```python
from build123d import *

# Parameters (mm, degrees)
SKETCH_1_W           = 40
SKETCH_1_H           = 45
EXTRUDE_1_DEPTH      = 40
EXTRUDE_1_DEPTH_BACK = 5
SKETCH_2_W           = 36
SKETCH_2_H           = 37
CUT_EXTRUDE_1_DEPTH  = 50
SKETCH_3_R           = 1.025
CUT_EXTRUDE_2_DEPTH  = 2
SKETCH_4_R           = 1.025
CUT_EXTRUDE_3_DEPTH  = 2
SKETCH_5_W           = 36
SKETCH_5_H           = 5
CUT_EXTRUDE_4_DEPTH  = 43
FILLET_6_R           = 5
FILLET_7_R           = 5


with BuildPart() as part:
    # 草圖1 → 填料-伸長1 (new body, two sides)
    with BuildSketch(Plane.XY) as extrude_1_sk:
        with Locations((5.454545455, -5.590909091)):
            Rectangle(SKETCH_1_W, SKETCH_1_H)
    extrude(amount=EXTRUDE_1_DEPTH)
    extrude(extrude_1_sk.sketch, amount=-EXTRUDE_1_DEPTH_BACK)

    # 草圖2 → 除料-伸長1 (cut)
    with BuildSketch(Plane(origin=(0, 16.909090909, 0), x_dir=(1, 0, 0), z_dir=(0, 1, 0))):
        with Locations((5.454545455, -21.5)):
            Rectangle(SKETCH_2_W, SKETCH_2_H)
    extrude(amount=-CUT_EXTRUDE_1_DEPTH, mode=Mode.SUBTRACT)

    # 草圖3 → 除料-伸長2 (cut)
    with BuildSketch(Plane.ZY.offset(14.545454545)):
        with Locations((37, -25.090909091)):
            Circle(SKETCH_3_R)
        with Locations((37, 13.909090909)):
            Circle(SKETCH_3_R)
    extrude(amount=-CUT_EXTRUDE_2_DEPTH, mode=Mode.SUBTRACT)

    # 草圖4 → 除料-伸長3 (cut)
    with BuildSketch(Plane(origin=(25.454545455, 0, 0), x_dir=(0, 0, -1), z_dir=(1, 0, 0))):
        with Locations((-37, 13.909090909)):
            Circle(SKETCH_4_R)
        with Locations((-37, -25.090909091)):
            Circle(SKETCH_4_R)
    extrude(amount=-CUT_EXTRUDE_3_DEPTH, mode=Mode.SUBTRACT)

    # 草圖5 → 除料-伸長4 (cut)
    with BuildSketch(Plane(origin=(0, 16.909090909, 0), x_dir=(1, 0, 0), z_dir=(0, 1, 0))):
        with Locations((5.454545455, -0.5)):
            Rectangle(SKETCH_5_W, SKETCH_5_H)
    extrude(amount=-CUT_EXTRUDE_4_DEPTH, mode=Mode.SUBTRACT)

    # 圓角6
    fillet_6_edges = [part.edges().sort_by_distance(p)[0] for p in [
        (-14.545454545, -5.590909091, -5),
    ]]
    fillet(fillet_6_edges, radius=FILLET_6_R)

    # 圓角7
    fillet_7_edges = [part.edges().sort_by_distance(p)[0] for p in [
        (25.454545455, -5.590909091, -5),
    ]]
    fillet(fillet_7_edges, radius=FILLET_7_R)


solid = part.part
```
Could you check a few things on this model? Use its own coordinates, in mm. A direction names the side the tool comes from. Round coordinates to 2 decimals unless told otherwise and drop trailing zeros. Write each loop counter-clockwise with the first axis right and the second up, starting at its lowest first coordinate (ties: lowest second). Pieces come first, ordered by that corner, then holes. Notation, with made-up numbers: M 36,12 L 89,12 A14 ccw 89,33 Z; hole C 68.25,-37.75 d1. An arc over 180 degrees is marked long. Write each question's results on one line, items separated by ' | '. Start each with the question number.
1. Thinking about a two-plate mould opening in Y: for faces 4 (the face through (24.469, 13.954, 38.024)), 5 (the face through (5.4, -28.091, 2.6)), 6 (the face through (5, -26.091, 0)), which applies, +Y half, -Y half, draft (parallel to the pull), parting line (faces both ways), or undercut?
2. On a 3-axis mill with a long thin cutter (end or side, diameter ignored), from which of +Z, -Z, +X, -X, +Y, -Y can I reach the whole of each face in a straight line? I mean faces 1 (the face through (5, -4, -2)), 2 (the face through (5, -27, 3)), 3 (the face through (-13.12, -5.276, -3.496)). Say none if no direction works.
3. Imagine slicing it at B-B on z = 24.5. List the corners of the cut face in (x, y) for me.
4. Imagine slicing it at A-A on z = 37. List the corners of the cut face in (x, y) for me, and give its area (3 significant figures).
5. Imagine slicing it at D-D on x = 12. List the corners of the cut face in (y, z) for me, and give its area (3 significant figures).
6. I'm going to push flat-ended pins straight in: pin 1 Ø1.8 at (y, z) = (-25.09, 37) entering from +X; pin 2 Ø2.5 at (x, z) = (12.5, 1.5) entering from +Y; pin 3 Ø3.5 at (y, z) = (13.91, 37) entering from +X; pin 4 Ø3 at (x, y) = (9.5, 1.5) entering from +Z. Where does each tip first touch, or does it pass through?
7. Imagine slicing it at C-C on y = 8. List the corners of the cut face in (x, z) for me.
8. I need wall thicknesses on L1, parallel to Y at x = 23.95, z = 37; L2, parallel to X at y = -13, z = 0.5; L3, parallel to Z at x = 14, y = -25.5. Which ranges of each line are inside material? Lowest first, please. Write a range as from..to.
Result sheet:
1) face 4: undercut | face 5: -Y half | face 6: +Y half
2) face 1: +Z, +Y | face 2: +Z, +Y, -Y | face 3: -Z, -X, +Y, -Y
3) outline: M -14.55,-28.09 L -12.55,-28.09 L -12.55,16.91 L -14.55,16.91 Z; M 23.45,-28.09 L 25.45,-28.09 L 25.45,16.91 L 23.45,16.91 Z
4) outline: M -14.55,-28.09 L -12.55,-28.09 L -12.55,-26.12 L -14.55,-26.12 Z; M -14.55,-24.07 L -12.55,-24.07 L -12.55,12.88 L -14.55,12.88 Z; M -14.55,14.93 L -12.55,14.93 L -12.55,16.91 L -14.55,16.91 Z; M 23.45,-28.09 L 25.45,-28.09 L 25.45,-26.12 L 23.45,-26.12 Z; M 23.45,-24.07 L 25.45,-24.07 L 25.45,12.88 L 23.45,12.88 Z; M 23.45,14.93 L 25.45,14.93 L 25.45,16.91 L 23.45,16.91 Z | area: 164 mm^2
5) outline: M -28.09,-5 L 16.91,-5 L 16.91,-2 L -26.09,-2 L -26.09,3 L -28.09,3 Z | area: 145 mm^2
6) pin 1: passes through | pin 2: stops at y = -26.09 | pin 3: stops at x = 25.45 | pin 4: stops at z = -2
7) outline: M -14.55,0 A5 ccw -9.55,-5 L 20.45,-5 A5 ccw 25.45,0 L 25.45,40 L 23.45,40 L 23.45,-2 L -12.55,-2 L -12.55,40 L -14.55,40 Z
8) L1: y = -28.09..-26.12, -24.07..12.88, 14.93..16.91 | L2: x = -14.55..-12.55, 23.45..25.45 | L3: z = -5..-2
